Read the model definition and answer for the solid it produces. Units are mm, in the model's axes. Face numbers are marked on the shaded views. A direction names the side the tool comes from. Give positions to 0.01 mm unless a question says otherwise; leave off trailing zeros. Write each loop counter-clockwise with the first axis right and the second up, starting at its lowest first coordinate (ties: lowest second). Pieces come first, ordered by that corner, then holes. Notation, with made-up numbers: (44.5, -7) -> (50.5, -7) arc R25 cw to (50.5, 18) -> close; hole circle Ø8 at (-24, 46.25). An arc over 180 degrees is marked (long way). Use a Markdown table: item, result.
from build123d import *

# Parameters (mm, degrees)
F0_R     = 43
F0_R_2   = 40
F1_DEPTH = 30
F2_DEPTH = 70
F0_R_3   = 1
F0_R_4   = 32.5
F3_DEPTH = 10
F4_R     = 43
F4_R_2   = 40
F4_R_3   = 5
F5_DEPTH = 3
F6_R     = 5


with BuildPart() as f1:
    # F0 (on Top) → F1 (new body)
    with BuildSketch(Plane.XY):
        Circle(F0_R)
        Circle(F0_R_2, mode=Mode.SUBTRACT)
    extrude(amount=F1_DEPTH)

    # F0 (on Top) → F2 (join)
    with BuildSketch(Plane.XY):
        Circle(F0_R)
        Circle(F0_R_2, mode=Mode.SUBTRACT)
    extrude(amount=-F2_DEPTH)

    # F0 (on Top) → F3 (join)
    with BuildSketch(Plane.XY):
        Circle(F0_R_2)
        with Locations((0, -36)):
            Circle(F0_R_3, mode=Mode.SUBTRACT)
        with Locations((-36, 0)):
            Circle(F0_R_3, mode=Mode.SUBTRACT)
        Circle(F0_R_4, mode=Mode.SUBTRACT)
        with Locations((36, 0)):
            Circle(F0_R_3, mode=Mode.SUBTRACT)
        with Locations((0, 36)):
            Circle(F0_R_3, mode=Mode.SUBTRACT)
    extrude(amount=-F3_DEPTH)

    # F4 (on face) → F5 (join)
    with BuildSketch(Plane(origin=(0, 0, -70), x_dir=(1, 0, 0), z_dir=(0, 0, -1))):
        Circle(F4_R)
        Circle(F4_R_2, mode=Mode.SUBTRACT)
        Circle(F4_R_2)
        Circle(F4_R_3, mode=Mode.SUBTRACT)
    extrude(amount=-F5_DEPTH)

    # F6
    f6_edges = [f1.edges().sort_by_distance(p)[0] for p in [
        (-43, 0, -70),
        (-40, 0, -67),
    ]]
    fillet(f6_edges, radius=F6_R)


solid = f1.part
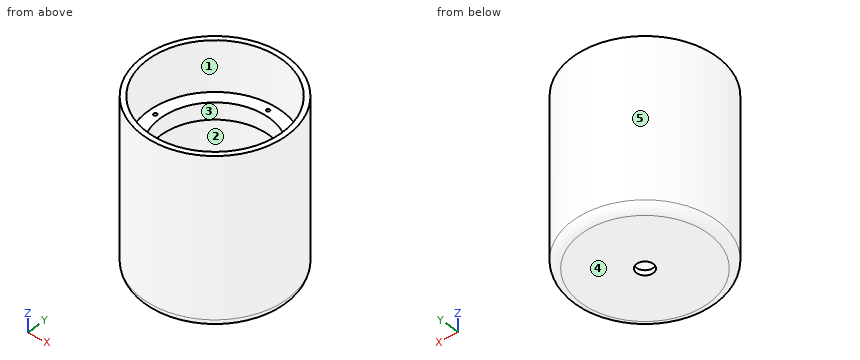
Item 1: A cutting plane is placed at A-A (z = -39.5). Give the vertices of the cut face in (x, y).
Return value:
| item | result |
|---|---|
| outline | circle Ø86 at (0, 0); hole circle Ø80 at (0, 0) |
Item 2: Straight lines are drawn through the part: line 1 along Y through (x, z) = (0, -36); line 2 along Z through (x, y) = (-21, 25); line 3 along X through (y, z) = (1, -55.5). For each, find the intervals that lie inside material, in ascending order. Write a range as [from, to].
Return value:
| item | result |
|---|---|
| line 1 | [-43, -40], [40, 43] |
| line 2 | [-70, -67], [-10, 0] |
| line 3 | [-42.99, -39.99], [39.99, 42.99] |
Item 3: A tool of negligible diameter and unlimited length cuts with its end or side. For the marked faces 1 and 2, from which of +Z, -Z, +X, -X, +Y, -Y can it reach the whole face along a straight path? Write none if from no direction.
Return value:
| item | result |
|---|---|
| face 1 | +Z |
| face 2 | none |
Item 4: Each of these flat-tipped pins is pushed along its axis until it touches: P1, Ø3, axis at x = -0.5, z = -3, coming from the -Y side; P2, Ø2.5, axis at x = -36, y = 0, coming from the +Z side; P3, Ø1.2, axis at x = 36, y = 0, coming from the +Z side. Where does it stop, or does it pass through?
Return value:
| item | result |
|---|---|
| P1 | y = -43 |
| P2 | z = 0 |
| P3 | z = -66.74 |
Item 5: For a pull along Y with two mould halves and no side action, classify the marked faces 3, 4 and 5 as +Y half, -Y half, draft (parallel to the pull), parting line (faces both ways), or undercut.
Return value:
| item | result |
|---|---|
| face 3 | undercut |
| face 4 | draft |
| face 5 | parting line |
